The listing builds one solid part. Answer for the finished solid, in the listing's coordinates (mm). Round coordinates to 2 decimals unless told otherwise and drop trailing zeros. Loops run counter-clockwise (first coordinate to the right, second up) from the corner with the lowest first, then second, coordinate; pieces in that order, holes last. Notation, with made-up numbers: M -16,55.25 L -3,55.25 A24 cw -3,69.25 Z; hole C 57.5,-9.75 d4. An arc over 180 degrees is marked long. Put each result on its own line as item: value. Start each with the question number.
(1) Section A-A, the plane x = 5.75 is taken. Determine the outline of the cut face in (y, z).
(2) Straight lines are drawn through the part: line 1 (X direction, y = 1.85, z = 6); line 2 (Z direction, x = 6, y = 0.3); line 3 (Z direction, x = -6.5, y = 1.1). For each, find the intervals that lie inside material, in ascending order.
(3) Section B-B, the plane y = 0.35 is taken. Count the separate pieces of the cut face and the enclosed holes in it, then the cut area to 3 significant figures.
(4) Section C-C, the plane x = -5.5 is taken. Determine the outline of the cut face in (y, z), then the cut area to 3 significant figures.
```python
from build123d import *

# Parameters (mm, degrees)
SKIZZE1_R                       = 7.4
AUFSATZ_LINEAR_AUSTRAGEN2_DEPTH = 2
SCHNITT_LINEAR_AUSTRAGEN2_DEPTH = 2


with BuildPart() as part:
    # Skizze1 → Aufsatz-Linear austragen2 (new body)
    with BuildSketch(Plane(origin=(0, 0, 0), x_dir=(1, 0, 0), z_dir=(0, 1, 0))):
        Circle(SKIZZE1_R)
    extrude(amount=AUFSATZ_LINEAR_AUSTRAGEN2_DEPTH)

    # Skizze3 → Schnitt-Linear austragen2 (cut)
    with BuildSketch(Plane.XZ):
        Polygon((3.110355434, 1.292281092), (3.433750851, 2.698961133), (2.377227909, 3.6823698), (0.99730955, 3.259098426), (0.673914133, 1.852418385), (1.730437075, 0.869009718), align=None)
        Polygon((1.051482334, -0.894820995), (1.374877751, 0.511859046), (0.318354809, 1.495267713), (-1.06156355, 1.071996339), (-1.384958967, -0.334683702), (-0.328436025, -1.318092369), align=None)
        Polygon((3.962790655, -1.57756505), (4.286186071, -0.170885009), (3.229663129, 0.812523658), (1.84974477, 0.389252284), (1.526349354, -1.017427757), (2.582872296, -2.000836424), align=None)
        Polygon((1.908536497, -3.73106102), (2.231931914, -2.324380979), (1.175408972, -1.340972312), (-0.204509387, -1.764243686), (-0.527904804, -3.170923727), (0.528618138, -4.154332394), align=None)
        Polygon((-0.967115848, -3.0562984), (-0.643720431, -1.649618359), (-1.700243373, -0.666209692), (-3.080161732, -1.089481066), (-3.403557149, -2.496161107), (-2.347034207, -3.479569774), align=None)
        Polygon((-1.811929532, -0.253503523), (-1.488534116, 1.153176518), (-2.545057058, 2.136585185), (-3.924975416, 1.713313811), (-4.248370833, 0.30663377), (-3.191847891, -0.676774897), align=None)
        Polygon((0.205432908, 1.896097632), (0.528828325, 3.302777673), (-0.527694618, 4.28618634), (-1.907612976, 3.862914966), (-2.231008393, 2.456234925), (-1.174485451, 1.472826258), align=None)
        Polygon((6.04694768, 0.660967687), (6.370343097, 2.067647728), (5.313820155, 3.051056395), (3.933901796, 2.627785021), (3.610506379, 1.22110498), (4.667029321, 0.237696313), align=None)
        Polygon((4.786465264, -4.469572088), (5.109860681, -3.062892047), (4.053337739, -2.07948338), (2.67341938, -2.502754754), (2.350023963, -3.909434795), (3.406546905, -4.892843462), align=None)
        Polygon((-0.16753074, -5.930350774), (0.155864677, -4.523670733), (-0.900658265, -3.540262066), (-2.280576624, -3.96353344), (-2.603972041, -5.370213481), (-1.547449099, -6.353622148), align=None)
        Polygon((-3.933901796, -2.438733427), (-3.610506379, -1.032053386), (-4.667029321, -0.048644719), (-6.04694768, -0.471916093), (-6.370343097, -1.878596134), (-5.313820155, -2.862004801), align=None)
        Polygon((-2.700371821, 2.561167603), (-2.376976404, 3.967847644), (-3.433499346, 4.951256311), (-4.813417705, 4.527984937), (-5.136813122, 3.121304896), (-4.08029018, 2.137896229), align=None)
        Polygon((2.26230049, 4.081327536), (2.585695906, 5.488007577), (1.529172964, 6.471416244), (0.149254605, 6.04814487), (-0.174140811, 4.641464829), (0.882382131, 3.658056162), align=None)
        Polygon((4.939265844, 3.431140862), (2.995205508, 5.228874076), (2.728936611, 4.059318245), (3.785459554, 3.075909578), align=None)
        Polygon((5.313820155, -2.556040794), (5.967525742, 0.044561799), (4.788744949, -0.337862256), (4.465349532, -1.744542297), align=None)
        Polygon((0.318354809, -5.813813764), (2.887600861, -5.054112189), (1.995209721, -4.223766537), (0.615291362, -4.647037911), align=None)
        Polygon((-3.042477939, -5.054112189), (-2.757057663, -3.831247126), (-3.813580605, -2.847838459), (-5.002736834, -3.209095193), align=None)
        Polygon((-4.766685593, 0.428469167), (-4.443290177, 1.835149208), (-5.251077368, 2.561167603), (-5.909694674, 0.044561799), align=None)
        Polygon((-0.667764964, 4.720679563), (-0.406041453, 5.906533391), (-2.986939248, 5.160492623), (-2.047683323, 4.297408189), align=None)
    extrude(amount=-SCHNITT_LINEAR_AUSTRAGEN2_DEPTH, mode=Mode.SUBTRACT)


solid = part.part
```
Recorded:
1. outline: M 0,-4.66 L 2,-4.66 L 2,-0.82 L 0,-0.82 Z; M 0,-0.03 L 2,-0.03 L 2,0.57 L 0,0.57 Z; M 0,2.65 L 2,2.65 L 2,4.66 L 0,4.66 Z
2. line 1: x = -4.33 to 0.14, 2.04 to 4.33
2. line 2: z = -4.33 to 0.65, 2.41 to 4.33
2. line 3: z = -3.54 to 3.54
3. separate pieces: 1
3. enclosed holes: 19
3. area: 88.8 mm²
4. outline: M 0,-4.95 L 2,-4.95 L 2,-2.69 L 0,-2.69 Z; M 0,-0.3 L 2,-0.3 L 2,0.18 L 0,0.18 Z; M 0,1.61 L 2,1.61 L 2,4.95 L 0,4.95 Z
4. area: 12.2 mm²
